Geometry check sheet. Reference: the model listing, model coordinates, mm. A direction names the side the tool comes from. Give positions to 0.01 mm unless a question says otherwise; leave off trailing zeros. Loops run counter-clockwise (first coordinate to the right, second up) from the corner with the lowest first, then second, coordinate; pieces in that order, holes last.
1. Cross-section at B-B, the plane z = -664. Record the cut outline in (x, y).
2. Go/stop test with flat-tipped pins: pin 1 Ø1 at (x, y) = (-597.5, 166) entering from -Z; pin 2 Ø4.5 at (x, z) = (-758.5, 111.5) entering from +Y; pin 3 Ø25 at (x, y) = (-25.5, 98.5) entering from -Z. Record where each tip stops, or that it passes through.
3. Cross-section at C-C, the plane y = 50.5. Record the cut outline in (x, z).
4. Release check for a two-part mould opening along Z. For faces 6 (the flat face through (-608, 412, 59.199)), 7 (the flat face through (-592, 413, 1009.199)), 8 (the flat face through (-1150, 412, 528)) record: +Z half, -Z half, draft (parallel to the pull), parting line (faces both ways), or undercut.
5. Tool access check on faces 1 (the flat face through (-25, 289, 109.199)), 2 (the flat face through (-50, 412, -473)), 3 (the flat face through (-608, 412, 959.199)), 4 (the flat face through (-608, -62.436, 84)), 5 (the flat face through (-25, 387.564, -458)). Record the directions out of +Z, -Z, +X, -X, +Y, -Y that give a thin tool (end or side, any length) a straight path to the whole face; none if there is none.
6. Material ranges on L1, parallel to Y at x = -847, z = 72; L2, parallel to Y at x = -195, z = 87; L3, parallel to X at y = 41.5, z = 110, recorded low to high.
7. Cross-section at A-A, the plane x = -136.5. Record the cut outline in (y, z), plus the area to 3 significant figures.
8. Cross-section at D-D, the plane y = 267. Record the cut outline in (x, z).
from build123d import *

# Parameters (mm, degrees)
F1_DEPTH  = 1200
F2_W      = 1100
F2_H      = 1050
F3_DEPTH  = 550.001
F4_W      = 1100
F4_H      = 850
F5_DEPTH  = 50.001
F6_R      = 5
F7_DEPTH  = 40
F8_W      = 1100
F8_H      = 450
F9_DEPTH  = 950.001
F10_W     = 1200
F10_H     = 300
F11_DEPTH = 4
F12_W     = 260
F12_H     = 130
F13_DEPTH = 4


with BuildPart() as f1:
    # F0 (on Right) → F1 (new body)
    with BuildSketch(Plane.YZ):
        Polygon((-112.436364, 109.19924), (-112.436364, -990.80076), (-62.436364, -990.80076), (-62.436364, 59.19924), (387.563636, 59.19924), (387.563636, -990.80076), (437.563636, -990.80076), (437.563636, 1009.19924), (387.563636, 1009.19924), (387.563636, 109.19924), align=None)
    extrude(amount=-F1_DEPTH)

    # F2 (on face) → F3 (cut, through all)
    with BuildSketch(Plane.XZ.offset(112.436364)):
        with Locations((-600, -465.80076)):
            Rectangle(F2_W, F2_H)
    extrude(amount=-F3_DEPTH, mode=Mode.SUBTRACT)

    # F4 (on face) → F5 (cut, through all)
    with BuildSketch(Plane.XZ.offset(-387.563636)):
        with Locations((-600, 534.19924)):
            Rectangle(F4_W, F4_H)
    extrude(amount=-F5_DEPTH, mode=Mode.SUBTRACT)

    # F6 (on face) → F7 (cut)
    with BuildSketch(Plane(origin=(0, 0, 59.19924), x_dir=(1, 0, 0), z_dir=(0, 0, -1))):
        with Locations((-847, 92.436364)):
            Circle(F6_R)
        with Locations((-353, 92.436364)):
            Circle(F6_R)
    extrude(amount=-F7_DEPTH, mode=Mode.SUBTRACT)

    # F8 (on face) → F9 (cut, through all)
    with BuildSketch(Plane(origin=(0, 0, 59.19924), x_dir=(1, 0, 0), z_dir=(0, 0, -1))):
        with Locations((-600, -162.563636)):
            Rectangle(F8_W, F8_H)
    extrude(amount=-F9_DEPTH, mode=Mode.SUBTRACT)

    # F10 (on face) → F11 (join)
    with BuildSketch(Plane.XY.offset(109.19924)):
        with Locations((-600, 37.563636)):
            Rectangle(F10_W, F10_H)
    extrude(amount=F11_DEPTH)

    # F12 (on face) → F13 (cut)
    with BuildSketch(Plane.XY.offset(113.19924)):
        with Locations((-600, 22.563636)):
            Rectangle(F12_W, F12_H)
    extrude(amount=-F13_DEPTH, mode=Mode.SUBTRACT)


solid = f1.part
Result:
1. outline: (-1200, -112.44) - (-1150, -112.44) - (-1150, -62.44) - (-1200, -62.44) - close; (-1200, 387.56) - (-1150, 387.56) - (-1150, 437.56) - (-1200, 437.56) - close; (-50, -112.44) - (0, -112.44) - (0, -62.44) - (-50, -62.44) - close; (-50, 387.56) - (0, 387.56) - (0, 437.56) - (-50, 437.56) - close
2. pin 1: stops at z = 109.2
2. pin 2: stops at y = 187.56
2. pin 3: stops at z = 59.2
3. outline: (-1200, 59.2) - (-1150, 59.2) - (-1150, 109.2) - (-730, 109.2) - (-730, 113.2) - (-1200, 113.2) - close; (-470, 109.2) - (-50, 109.2) - (-50, 59.2) - (0, 59.2) - (0, 113.2) - (-470, 113.2) - close
4. face 6: -Z half
4. face 7: +Z half
4. face 8: undercut
5. face 1: +Z, +X, -X
5. face 2: -Z, +Y, -Y
5. face 3: +Y, -Y
5. face 4: -Z
5. face 5: -Z, +X, -X
6. L1: y = -112.44 to -97.44, -87.44 to -62.44, 387.56 to 437.56
6. L2: y = -112.44 to -62.44, 387.56 to 437.56
6. L3: x = -1200 to -730, -470 to 0
7. outline: (-112.44, 59.2) - (-62.44, 59.2) - (-62.44, 109.2) - (187.56, 109.2) - (187.56, 113.2) - (-112.44, 113.2) - close; (387.56, 59.2) - (437.56, 59.2) - (437.56, 109.2) - (387.56, 109.2) - close; (387.56, 959.2) - (437.56, 959.2) - (437.56, 1009.2) - (387.56, 1009.2) - close
7. area: 8,700 mm2
8. outline: (-1200, 59.2) - (-1150, 59.2) - (-1150, 109.2) - (-1200, 109.2) - close; (-50, 59.2) - (0, 59.2) - (0, 109.2) - (-50, 109.2) - close
